```python
from build123d import *

# Parameters (mm, degrees)
BOSS_EXTRUDE1_DEPTH                                 = 12.7
CUT_EXTRUDE1_DEPTH                                  = 13.7
HOLE1_D                                             = 9
HOLE1_DEPTH                                         = 12.7
F_4_CLEARANCE_HOLE1_D                               = 3.3
F_4_CLEARANCE_HOLE1_DEPTH                           = 12.7
HOLE2_D                                             = 51
HOLE2_DEPTH                                         = 12.7
HOLE2_CBORE_D                                       = 88.9
HOLE2_CBORE_DEPTH                                   = 4
CBORE_FOR_8_BINDING_HEAD_MACHINE_SCREW1_D           = 4.5
CBORE_FOR_8_BINDING_HEAD_MACHINE_SCREW1_DEPTH       = 12.7
CBORE_FOR_8_BINDING_HEAD_MACHINE_SCREW1_CBORE_D     = 8.25
CBORE_FOR_8_BINDING_HEAD_MACHINE_SCREW1_CBORE_DEPTH = 4
FILLET1_R                                           = 10
SKETCH11_R                                          = 2
CUT_EXTRUDE2_DEPTH                                  = 13.7


with BuildPart() as part:
    # Sketch1 → Boss-Extrude1 (new body)
    with BuildSketch(Plane.XY.offset(12.7)):
        with BuildLine():
            Line((40, -170), (73.308387301, -15.839202988))
            ThreePointArc((73.308387301, -15.839202988), (0, 75), (-73.308387301, -15.839202988))
            Line((-73.308387301, -15.839202988), (-40, -170))
            Line((-40, -170), (40, -170))
        make_face()
    extrude(amount=-BOSS_EXTRUDE1_DEPTH)

    # Sketch2 → Cut-Extrude1 (cut, through all)
    with BuildSketch(Plane(origin=(0, 0, 0), x_dir=(-1, 0, 0), z_dir=(0, 0, -1))):
        with BuildLine():
            Line((-18.5, -124), (-18.5, -134))
            ThreePointArc((-18.5, -134), (0, -152.5), (18.5, -134))
            Line((18.5, -134), (18.5, -124))
            ThreePointArc((18.5, -124), (0, -105.5), (-18.5, -124))
        make_face()
    extrude(amount=-CUT_EXTRUDE1_DEPTH, mode=Mode.SUBTRACT)

    # Hole1
    with Locations(Plane(origin=(0, 0, 0), x_dir=(-1, 0, 0), z_dir=(0, 0, -1))):
        with Locations((-50, -60), (50, -60), (50, 40), (-50, 40)):
            Hole(HOLE1_D / 2, depth=HOLE1_DEPTH)

    # #4 Clearance Hole1
    with Locations(Plane.XY.offset(12.7)):
        with Locations((-31.929873349, -160), (-25.5, -116.75), (-25.5, -141.25), (25.5, -116.75), (25.5, -141.25)):
            Hole(F_4_CLEARANCE_HOLE1_D / 2, depth=F_4_CLEARANCE_HOLE1_DEPTH)

    # Hole2
    with Locations(Plane.XY.offset(12.7)):
        with Locations((0, 0)):
            CounterBoreHole(HOLE2_D / 2, HOLE2_CBORE_D / 2, HOLE2_CBORE_DEPTH, depth=HOLE2_DEPTH)

    # CBORE for #8 Binding Head Machine Screw1
    with Locations(Plane(origin=(0, 0, 0), x_dir=(-1, 0, 0), z_dir=(0, 0, -1))):
        with Locations((28.991378029, 28.991378029), (41, 0), (28.991378029, -28.991378029), (0, -41), (-28.991378029, -28.991378029), (-41, 0), (-28.991378029, 28.991378029), (0, 41)):
            CounterBoreHole(CBORE_FOR_8_BINDING_HEAD_MACHINE_SCREW1_D / 2, CBORE_FOR_8_BINDING_HEAD_MACHINE_SCREW1_CBORE_D / 2, CBORE_FOR_8_BINDING_HEAD_MACHINE_SCREW1_CBORE_DEPTH, depth=CBORE_FOR_8_BINDING_HEAD_MACHINE_SCREW1_DEPTH)

    # Fillet1
    fillet1_edges = [part.edges().sort_by_distance(p)[0] for p in [
        (-40, -170, 6.35),
        (40, -170, 6.35),
    ]]
    fillet(fillet1_edges, radius=FILLET1_R)

    # Sketch11 → Cut-Extrude2 (cut, through all)
    with BuildSketch(Plane.XY.offset(12.7)):
        with Locations((-70, 0)):
            Circle(SKETCH11_R)
        with Locations((70, 0)):
            Circle(SKETCH11_R)
    extrude(amount=-CUT_EXTRUDE2_DEPTH, mode=Mode.SUBTRACT)


solid = part.part
```
Input: part model. Units: mm. Frame: model coordinates. A direction names the side the tool comes from. Coordinates: 2 decimals unless noted, no trailing zeros. Write each loop counter-clockwise with the first axis right and the second up, starting at its lowest first coordinate (ties: lowest second). Pieces come first, ordered by that corner, then holes.
1) Section A-A on x = -50. Output: boundary loops of the cut face in (y, z), and give its area (3 significant figures).
2) Set-up query: faces 5 (the flat face through (18.5, -129, 6)), 6 (the cylindrical face through (27.09, -32.65, 1.97)), 7 (the cylindrical face through (42.397, 13.352, 10.728)). Return all of +Z, -Z, +X, -X, +Y, -Y with unobstructed straight access to the full face (end or side cutting, diameter ignored); none if empty.
3) Pin query (flat end, axial travel): pin 1 Ø7 at (x, y) = (-28.99, 28.99) entering from -Z; pin 2 Ø14.5 at (x, y) = (50, -60) entering from -Z; pin 3 Ø1 at (y, z) = (-49.5, 9.5) entering from +X; pin 4 Ø1.5 at (y, z) = (-87, 5.5) entering from -X. Return the tip coordinate at first contact, or that it passes through.
4) Material intervals for line 1 along Y through (x, z) = (2, 12); line 2 along Y through (x, z) = (-12, 4); line 3 along X through (y, z) = (30.5, 1.5), sorted ascending.
5) Section B-B on y = 21. Output: boundary loops of the cut face in (x, z), and give its area (3 significant figures).
6) Mould query, pull axis X, two halves, no side actions, for faces 1 (the cylindrical face through (-0.407, -105.504, 6.261)), 2 (the cylindrical face through (45.12, 0.18, 1.97)), 3 (the flat face through (-1, -46, 12.7)), 4 (the cylindrical face through (-38.14, -167.84, 6.26)). Classes: pulls with the +X half, pulls with the -X half, needs draft (parallel to the pull), parting line crosses it, or undercut.
Check result:
1. outline: (-123.72, 0) - (-64.5, 0) - (-64.5, 12.7) - (-123.72, 12.7) - close; (-55.5, 0) - (35.5, 0) - (35.5, 12.7) - (-55.5, 12.7) - close; (44.5, 0) - (55.9, 0) - (55.9, 12.7) - (44.5, 12.7) - close
1. area: 2,050 mm2
2. face 5: +Z, -Z
2. face 6: -Z
2. face 7: +Z
3. pin 1: stops at z = 4
3. pin 2: stops at z = 0
3. pin 3: stops at x = 66.14
3. pin 4: stops at x = -58.1
4. line 1: y = -170 to -152.39, -105.61 to -44.4, 44.4 to 74.97
4. line 2: y = -170 to -148.08, -109.92 to -22.5, 22.5 to 74.03
4. line 3: x = -68.52 to -32.83, -25.15 to 25.15, 32.83 to 68.52
5. outline: (-72, 0) - (-14.47, 0) - (-14.47, 8.7) - (-39.18, 8.7) - (-39.18, 12.7) - (-72, 12.7) - close; (14.47, 0) - (72, 0) - (72, 12.7) - (39.18, 12.7) - (39.18, 8.7) - (14.47, 8.7) - close
5. area: 1,260 mm2
6. face 1: undercut
6. face 2: undercut
6. face 3: needs draft
6. face 4: pulls with the -X half
